Autodesk Fusion 360 part; units mm, degrees
sketch "Schizzo1" plane through (0, 0, 0) normal (0, 0, 1) x (1, 0, 0)
  line L0 (0, 0) -> (-25, 0)
  line L1 (-25, 0) -> (-25, 3)
  line L2 (-25, 3) -> (-5, 3)
  line L3 (-5, 3) -> (-5, 11.5)
  line L4 (-5, 11.5) -> (-25, 11.5)
  line L5 (-25, 11.5) -> (-25, 14.5)
  line L6 (-25, 14.5) -> (0, 14.5)
  line L7 (0, 14.5) -> (0, 0)
  line L8 (10.253, 10.253) -> (27.9307, -7.4246)
  line L9 (11.6673, 4.5962) -> (5.6569, -1.4142)
  line L10 (0, 0) -> (10.253, 10.253)
  line L11 (17.6777, -17.6777) -> (0, 0)
  line L12 (5.6569, -1.4142) -> (19.799, -15.5563)
  line L13 (27.9307, -7.4246) -> (25.8094, -9.5459)
  line L14 (19.799, -15.5563) -> (17.6777, -17.6777)
  line L15 (25.8094, -9.5459) -> (11.6673, 4.5962)
  line L16 (0, 14.5) -> (10.253, 10.253)
  point P0 (10.253, 10.253)
  dimension "d2" = 8.5
  dimension "d3" = 3
  dimension "d4" = 3
  dimension "d5" = 25
  dimension "d6" = 25
  dimension "d7" = 20
  dimension "d8" = 8.5
  dimension "d9" = 3
  dimension "d10" = 3
  dimension "d11" = 25
  dimension "d12" = 25
  dimension "d13" = 20
  dimension "d16" = 45
extrude "Estrusione1" add sketch "Schizzo1" along normal blind 250
fillet "Raccordo1" radius 5 1 edges at (0, 0, 125)
Verification items for the finished model (mm, model axes). A direction names the side the tool comes from. Round coordinates to 2 decimals unless told otherwise and drop trailing zeros. Write each loop counter-clockwise with the first axis right and the second up, starting at its lowest first coordinate (ties: lowest second). Pieces come first, ordered by that corner, then holes. Notation, with made-up numbers: (-27.75, 32.25) - (14.25, 32.25) arc R29 ccw to (14.25, 57.25) - close; hole circle Ø7 at (-12, 54). An arc over 180 degrees is marked (long way). Answer as a JSON object with one key per item and string values. Group by question number.
Q1. Mould release check, pull along X, two halves, no side actions. Record for faces 1 (the flat face through (18.837, -2.574, 123.25)), 2 (the flat face through (-15, 11.5, 123)), 3 (the flat face through (18.968, 1.538, 123.25)), 4 (the flat face through (10, -10, 123)): released by +X, released by -X, zero draft, split by the parting line, or undercut.
Q2. Section check A-A, the plane x = -20. Enter the section's corners in (y, z), plus the area to 3 significant figures.
Q3. Tool access check on faces 5 (the flat face through (1, 4, 250)), 6 (the flat face through (-13, 0, 123)), 7 (the flat face through (-5, 7, 123)), 8 (the flat face through (12.63, -8.39, 123.25)). Record the directions out of +Z, -Z, +X, -X, +Y, -Y that give a thin tool (end or side, any length) a straight path to the whole face; none if there is none.
Q4. Section check C-C, the plane y = -13. Enter the section's corners in (x, z), plus the area to 3 significant figures.
Q5. Thickness scan on line 1 (Y direction, x = -17.5, z = 186.5); line 2 (X direction, y = -9, z = 198); line 3 (X direction, y = -1.5, z = 44). Record the ranges inside material, lowest first.
Q6. Section check B-B, the plane z = 132. Enter the section's corners in (x, y), plus the area to 3 significant figures.
Q7. Go/stop test with flat-tipped pins: pin 1 Ø3 at (y, z) = (9, 155) entering from -X; pin 2 Ø25 at (x, z) = (-10, 126) entering from -Y; pin 3 Ø22 at (x, z) = (-20, 114.5) entering from -Y. Record where each tip stops, or that it passes through.
Found:
{
 "1": {"face 1": "undercut", "face 2": "zero draft", "face 3": "released by +X", "face 4": "released by -X"},
 "2": {"outline": "(0, 0) - (3, 0) - (3, 250) - (0, 250) - close; (11.5, 0) - (14.5, 0) - (14.5, 250) - (11.5, 250) - close", "area": "1,500 mm^2"},
 "3": {"face 5": "+Z, +X, -X, +Y, -Y", "face 6": "+Z, -Z, -X, -Y", "face 7": "+Z, -Z, -X", "face 8": "+Z, -Z"},
 "4": {"outline": "(13, 0) - (17.24, 0) - (17.24, 250) - (13, 250) - close", "area": "1,060 mm^2"},
 "5": {"line 1": "y = 0 to 3, 11.5 to 14.5", "line 2": "x = 9 to 13.24, 25.26 to 26.36", "line 3": "x = 1.5 to 5.74, 17.76 to 22.01"},
 "6": {"outline": "(-25, 0) - (-2.07, 0) arc R5 cw to (1.46, -1.46) - (17.68, -17.68) - (19.8, -15.56) - (5.66, -1.41) - (11.67, 4.6) - (25.81, -9.55) - (27.93, -7.42) - (10.25, 10.25) - (0, 14.5) - (-25, 14.5) - (-25, 11.5) - (-5, 11.5) - (-5, 3) - (-25, 3) - close", "area": "460 mm^2"},
 "7": {"pin 1": "stops at x = -5", "pin 2": "stops at y = -2.5", "pin 3": "stops at y = 0"}
}
